Geometry: final body of the model. Coordinates: model frame, mm. Give positions to 0.01 mm unless a question says otherwise; leave off trailing zeros. Order: outer loops, then holes, each group sorted by start corner. A loop starts at its lowest first (then second) coordinate and runs counter-clockwise, first axis right, second up. Notation, with made-up numbers: (75, -3.75) -> (121, -3.75) arc R12 ccw to (121, 1.25) -> close; hole circle Ø9 at (7.25, 44). An arc over 180 degrees is marked (long way). Write item = value, one per line.
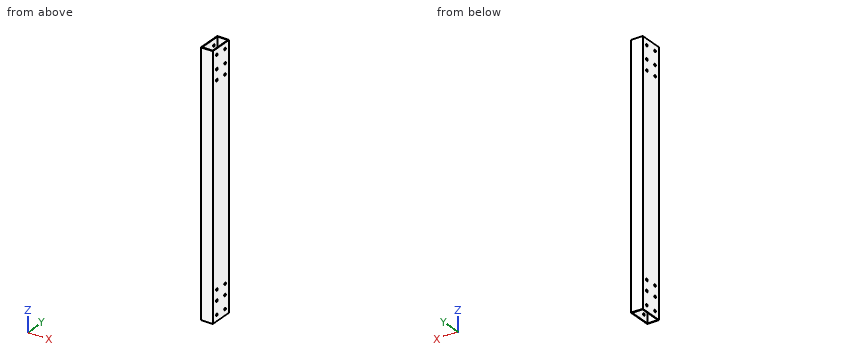
```python
from build123d import *

# Parameters (mm, degrees)
SKETCH1_W           = 25.4
SKETCH1_H           = 50.8
SKETCH1_W_2         = 22.225
SKETCH1_H_2         = 47.625
BOSS_EXTRUDE1_DEPTH = 546.1
SKETCH2_R           = 2.54
CUT_EXTRUDE1_DEPTH  = 550.045544559


with BuildPart() as part:
    # Sketch1 → Boss-Extrude1 (new body)
    with BuildSketch(Plane.XY):
        with Locations((12.7, 25.4)):
            Rectangle(SKETCH1_W, SKETCH1_H)
        with Locations((12.7, 25.4)):
            Rectangle(SKETCH1_W_2, SKETCH1_H_2, mode=Mode.SUBTRACT)
    extrude(amount=BOSS_EXTRUDE1_DEPTH)

    # Sketch2 → Cut-Extrude1 (cut, through all)
    with BuildSketch(Plane(origin=(25.4, 0, 0), x_dir=(0, 0, -1), z_dir=(1, 0, 0))):
        with Locations((-504.825, 38.1)):
            Circle(SKETCH2_R)
        with Locations((-504.825, 12.7)):
            Circle(SKETCH2_R)
        with Locations((-482.6, 38.1)):
            Circle(SKETCH2_R)
        with Locations((-482.6, 12.7)):
            Circle(SKETCH2_R)
        with Locations((-533.4, 12.7)):
            Circle(SKETCH2_R)
        with Locations((-533.4, 38.1)):
            Circle(SKETCH2_R)
        with Locations(Location((-12.7, 38.1, 0), (0, 0, 180))):
            Circle(SKETCH2_R)
        with Locations(Location((-12.7, 12.7, 0), (0, 0, 180))):
            Circle(SKETCH2_R)
        with Locations(Location((-63.5, 12.7, 0), (0, 0, 180))):
            Circle(SKETCH2_R)
        with Locations(Location((-63.5, 38.1, 0), (0, 0, 180))):
            Circle(SKETCH2_R)
        with Locations(Location((-41.275, 12.7, 0), (0, 0, 180))):
            Circle(SKETCH2_R)
        with Locations(Location((-41.275, 38.1, 0), (0, 0, 180))):
            Circle(SKETCH2_R)
    extrude(amount=-CUT_EXTRUDE1_DEPTH, mode=Mode.SUBTRACT)


solid = part.part
```
1) Section query A-A (x = 5.5). Output: boundary loops of the cut face in (y, z), plus the area to 3 significant figures.
Check sheet entries:
outline = (0, 0) -> (1.59, 0) -> (1.59, 546.1) -> (0, 546.1) -> close; (49.21, 0) -> (50.8, 0) -> (50.8, 546.1) -> (49.21, 546.1) -> close
area = 1,730 mm²
2) Line query: line 1 (Y direction, x = 25.05, z = 12.7); line 2 (X direction, y = 39.5, z = 332.5); line 3 (Y direction, x = 7, z = 435.5). Output: solid intervals per line, ascending. Write a range as from..to.
Check sheet entries:
line_1 = 0..10.16, 15.24..35.56, 40.64..50.8
line_2 = 0..1.59, 23.81..25.4
line_3 = 0..1.59, 49.21..50.8
3) First-contact query: P1, Ø6, axis at y = 38.1, z = 41.275, coming from the -X side. Flat tip, straight axial feed; report the tip coordinate or a pass-through.
Check sheet entries:
P1 = 0
4) Section query B-B (z = 329). Output: boundary loops of the cut face in (x, y), plus the area to 3 significant figures.
Check sheet entries:
outline = (0, 0) -> (25.4, 0) -> (25.4, 50.8) -> (0, 50.8) -> close; hole (1.59, 1.59) -> (23.81, 1.59) -> (23.81, 49.21) -> (1.59, 49.21) -> close
area = 232 mm²
